```python
from build123d import *

# Parameters (mm, degrees)
SKETCH2_R                = 2.5
BOSS_EXTRUDE1_DEPTH      = 4
BOSS_EXTRUDE2_DEPTH      = 4
BOSS_EXTRUDE2_DEPTH_BACK = 4
BOSS_EXTRUDE3_REACH      = 138.997
BOSS_EXTRUDE3_END_RADIUS = 14
SKETCH4_W                = 8
SKETCH4_H                = 8
SKETCH5_R                = 5.4
CUT_EXTRUDE1_DEPTH       = 0.5


with BuildPart() as part:
    # Sketch2 → Boss-Extrude1 (new body)
    with BuildSketch(Plane(origin=(0, 0, 0), x_dir=(1, 0, 0), z_dir=(0, 1, 0))):
        with BuildLine():
            Line((-126.75, 7.5), (31.75, 7.5))
            ThreePointArc((31.75, 7.5), (39.25, 0), (31.75, -7.5))
            Line((31.75, -7.5), (-126.75, -7.5))
            ThreePointArc((-126.75, -7.5), (-134.25, 0), (-126.75, 7.5))
        make_face()
        with Locations(Location((-31.75, 0, 0), (0, 0, 270))):
            Circle(SKETCH2_R, mode=Mode.SUBTRACT)
        with Locations(Location((31.75, 0, 0), (0, 0, 270))):
            Circle(SKETCH2_R, mode=Mode.SUBTRACT)
    extrude(amount=BOSS_EXTRUDE1_DEPTH)



with BuildPart() as body_2:
    # Sketch3 → Boss-Extrude2 (new, two sides: drawn at the far end of the back side and taken through both)
    with BuildSketch(Plane(origin=(-125, 0, 0), x_dir=(0, 0, -1), z_dir=(1, 0, 0)).offset(-BOSS_EXTRUDE2_DEPTH_BACK)):
        with BuildLine():
            Line((-13.787308542, 27.431074487), (-11.32528916, 26.996954043))
            ThreePointArc((-11.32528916, 26.996954043), (0, 13.5), (11.32528916, 26.996954043))
            Line((11.32528916, 26.996954043), (13.787308542, 27.431074487))
            ThreePointArc((13.787308542, 27.431074487), (0, 11), (-13.787308542, 27.431074487))
        make_face()
    extrude(amount=BOSS_EXTRUDE2_DEPTH + BOSS_EXTRUDE2_DEPTH_BACK)


with BuildPart() as part_1:
    add(part.part)

    add(body_2.part)  # Boss-Extrude3 merges body 2
    # Boss-Extrude3: up to this cylinder (the profile starts outside it)
    boss_extrude3_end = Plane(origin=(-125, 25, 0), z_dir=(1, 0, 0)) * Cylinder(BOSS_EXTRUDE3_END_RADIUS, 306.994, mode=Mode.PRIVATE)
    # Sketch4 → Boss-Extrude3 (add, up to the surface)
    with BuildSketch(Plane(origin=(0, 4, 0), x_dir=(1, 0, 0), z_dir=(0, 1, 0)), mode=Mode.PRIVATE) as boss_extrude3_sk1:
        with Locations((-125, 0)):
            Rectangle(SKETCH4_W, SKETCH4_H)
    boss_extrude3_tool1 = extrude(boss_extrude3_sk1.sketch, amount=BOSS_EXTRUDE3_REACH, mode=Mode.PRIVATE) - boss_extrude3_end
    add(boss_extrude3_tool1.solids().sort_by_distance((-125, 4, 0))[0])

    # Sketch5 → Cut-Extrude1 (cut)
    with BuildSketch(Plane.XZ):
        with Locations(Location((-31.75, 0, 0), (0, 0, 270))):
            Circle(SKETCH5_R)
        with Locations(Location((31.75, 0, 0), (0, 0, 270))):
            Circle(SKETCH5_R)
    extrude(amount=-CUT_EXTRUDE1_DEPTH, mode=Mode.SUBTRACT)


solid = part_1.part
```
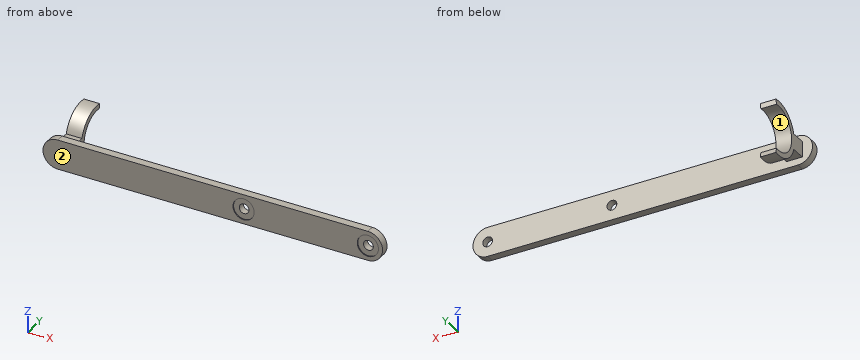
Source: CAD feature listing. Evaluate the final solid. Frame: model axes, mm. Face numbers are marked on the shaded views. Give positions to 0.01 mm unless a question says otherwise; leave off trailing zeros. Loops run counter-clockwise (first coordinate to the right, second up) from the corner with the lowest first, then second, coordinate; pieces in that order, holes last. Notation, with made-up numbers: (16.25, 46.5) - (22.25, 46.5) arc R23 cw to (22.25, 69.5) - close; hole circle Ø4 at (11, -26). An arc over 180 degrees is marked (long way). Use CSV: the item, a comma, the result in double quotes. Start each with the question number.
1. Ray query, L1, parallel to X at y = 1.55, z = 0; L2, parallel to X at y = 0.25, z = 0; L3, parallel to Z at x = 31.75, y = 2.15. Return the intervals inside material, ascending.
2. Pin query (flat end, axial travel): pin 1 (16.5 mm diameter, centred on x = -42.5, z = -2, fed in from +Y); pin 2 (4 mm diameter, centred on x = -124.5, y = 9.5, fed in from +Z); pin 3 (1 mm diameter, centred on x = -74.5, z = -2.5, fed in from -Y); pin 4 (4.5 mm diameter, centred on x = -78, y = 1.5, fed in from -Z). Return the tip coordinate at first contact, or that it passes through.
3. Section B-B (y = 25). Output: boundary loops of the cut face in (x, z).
4. Draft query along Y for the marked faces 1 and 2. Return one class per face: +Y half, -Y half, draft (parallel to the pull), parting line (faces both ways), or undercut.
5. Section A-A (x = -31.75). Output: boundary loops of the cut face in (y, z), then the cut area to 3 significant figures.
6. Section C-C (z = 0). Output: boundary loops of the cut face in (x, y).
7. Section D-D (y = 2.5). Output: boundary loops of the cut face in (x, z).
Response:
1,L1,"-134.25 to -34.25, -29.25 to 29.25, 34.25 to 39.25"
1,L2,"-134.25 to -37.15, -26.35 to 26.35, 37.15 to 39.25"
1,L3,"-7.5 to -2.5, 2.5 to 7.5"
2,pin 1,"y = 4"
2,pin 2,"z = 4"
2,pin 3,"y = 0"
2,pin 4,"z = -7.5"
3,outline,"(-129, -14) - (-121, -14) - (-121, -11.5) - (-129, -11.5) - close; (-129, 11.5) - (-121, 11.5) - (-121, 14) - (-129, 14) - close"
4,face 1,"undercut"
4,face 2,"-Y half"
5,outline,"(0, -7.5) - (4, -7.5) - (4, -2.5) - (0.5, -2.5) - (0.5, -5.4) - (0, -5.4) - close; (0, 5.4) - (0.5, 5.4) - (0.5, 2.5) - (4, 2.5) - (4, 7.5) - (0, 7.5) - close"
5,area,"37.1 mm²"
6,outline,"(-134.25, 0) - (-37.15, 0) - (-37.15, 0.5) - (-34.25, 0.5) - (-34.25, 4) - (-121, 4) - (-121, 13.5) - (-129, 13.5) - (-129, 4) - (-134.25, 4) - close; (-29.25, 0.5) - (-26.35, 0.5) - (-26.35, 0) - (26.35, 0) - (26.35, 0.5) - (29.25, 0.5) - (29.25, 4) - (-29.25, 4) - close; (34.25, 0.5) - (37.15, 0.5) - (37.15, 0) - (39.25, 0) - (39.25, 4) - (34.25, 4) - close"
7,outline,"(-126.75, -7.5) - (31.75, -7.5) arc R7.5 ccw to (31.75, 7.5) - (-126.75, 7.5) arc R7.5 ccw to start; hole circle Ø5 at (-31.75, 0); hole circle Ø5 at (31.75, 0)"
